```python
from build123d import *

# Parameters (mm, degrees)
SALIENTE_EXTRUIR2_DEPTH = 0.1
SALIENTE_EXTRUIR3_DEPTH = 0.1


with BuildPart() as part:
    # Croquis1 → Saliente-Extruir2 (new body)
    with BuildSketch(Plane.XY):
        with BuildLine():
            Line((-47.708333333, 74.739583333), (62.291666667, 74.739583333))
            ThreePointArc((62.291666667, 74.739583333), (76.43380229, 68.881718957), (82.291666667, 54.739583333))
            Line((82.291666667, 54.739583333), (82.291666667, -85.260416667))
            ThreePointArc((82.291666667, -85.260416667), (76.43380229, -99.40255229), (62.291666667, -105.260416667))
            Line((62.291666667, -105.260416667), (-47.708333333, -105.260416667))
            ThreePointArc((-47.708333333, -105.260416667), (-61.850468957, -99.40255229), (-67.708333333, -85.260416667))
            Line((-67.708333333, -85.260416667), (-67.708333333, 54.739583333))
            ThreePointArc((-67.708333333, 54.739583333), (-61.850468957, 68.881718957), (-47.708333333, 74.739583333))
        make_face()
    extrude(amount=SALIENTE_EXTRUIR2_DEPTH)

    # Croquis2 → Saliente-Extruir3 (add)
    with BuildSketch(Plane.XY.offset(0.1)):
        Polygon((-32.708333333, -55.260416667), (7.291666667, 34.739583333), (47.291666667, -55.260416667), align=None)
    extrude(amount=SALIENTE_EXTRUIR3_DEPTH)


solid = part.part
```
Check sheet for the modelled part. Datum: model origin and axes. Units: mm. Give positions to 0.01 mm unless a question says otherwise; leave off trailing zeros. Write each loop counter-clockwise with the first axis right and the second up, starting at its lowest first coordinate (ties: lowest second). Pieces come first, ordered by that corner, then holes.
Item 1: Cross-section at C-C (x = -35). Enter the section's corners in (y, z).
Item 2: Cross-section at A-A (x = -13.5). Enter the section's corners in (y, z).
Item 3: Cross-section at B-B (y = 28). Enter the section's corners in (x, z).
Item 4: Cross-section at D-D (y = 46). Enter the section's corners in (x, z).
Item 5: Gauge pin test, flat end, axial feed: pin 1 (1 mm diameter, centred on x = -38, y = -10, fed in from +Z). Record the tip position at first contact, or that the pin passes through.
Item 6: Scan lines: L1, parallel to X at y = -22, z = 0.15; L2, parallel to Y at x = -31.5, z = 0.15; L3, parallel to Y at x = 14.5, z = 0.15. Record each from-to range of solid material in increasing order.
Report:
1. outline: (-105.26, 0) - (74.74, 0) - (74.74, 0.1) - (-105.26, 0.1) - close
2. outline: (-105.26, 0) - (74.74, 0) - (74.74, 0.1) - (-12.04, 0.1) - (-12.04, 0.2) - (-55.26, 0.2) - (-55.26, 0.1) - (-105.26, 0.1) - close
3. outline: (-67.71, 0) - (82.29, 0) - (82.29, 0.1) - (10.29, 0.1) - (10.29, 0.2) - (4.3, 0.2) - (4.3, 0.1) - (-67.71, 0.1) - close
4. outline: (-67.71, 0) - (82.29, 0) - (82.29, 0.1) - (-67.71, 0.1) - close
5. pin 1: stops at z = 0.1
6. L1: x = -17.93 to 32.51
6. L2: y = -55.26 to -52.54
6. L3: y = -55.26 to 18.52
